Autodesk Inventor part; units mm, degrees
ref_plane "YZ Plane" through (0, 0, 0) normal (1, 0, 0) x (0, 1, 0)
ref_plane "XZ Plane" through (0, 0, 0) normal (0, 1, 0) x (-1, 0, 0)
ref_plane "XY Plane" through (0, 0, 0) normal (0, 0, 1) x (1, 0, 0)
sketch "Sketch1" plane through (0, 0, 0) normal (0, 1, 0) x (-1, 0, 0)
  line L0 (32.5791, 64.9096) -> (-50.4209, 64.9096)
  line L1 (-50.4209, 64.9096) -> (-50.4209, -78.0904)
  line L2 (-50.4209, -78.0904) -> (32.5791, -78.0904)
  line L3 (32.5791, -78.0904) -> (32.5791, 64.9096)
  line L4 (29.5791, 61.9096) -> (-47.4209, 61.9096)
  line L5 (-47.4209, 61.9096) -> (-47.4209, -75.0904)
  line L6 (-47.4209, -75.0904) -> (29.5791, -75.0904)
  line L7 (29.5791, -75.0904) -> (29.5791, 61.9096)
  line L8 (29.5791, -75.0904) -> (29.5791, -78.0904)
  line L9 (-47.4209, -70.2006) -> (-50.4209, -70.2006)
  line L10 (-47.4209, 33.4969) -> (-50.4209, 33.4969)
  line L11 (29.5791, 57.9608) -> (32.5791, 57.9608)
  line L12 (29.5791, -75.0904) -> (32.5791, -75.0904)
  point P0 (0, 0)
  dimension "d0" = 143
  dimension "d1" = 83
  dimension "d2" = 3
extrude "Floor" add sketch "Sketch1" along normal blind 3
extrude "Walls" add sketch "Sketch1" along normal blind 20 contours L3 L11 L7 L4 L5 L10 L1 L0 | L3 L12 L7 L11 | L10 L5 L9 L1 | L3 L2 L8 L12 | L9 L5 L6 L8 L2 L1
sketch "Sketch2" plane through (0, 0, 0) normal (0, 1, 0) x (-1, 0, 0)
  line L0 (-47.4209, 61.9096) -> (29.5791, 61.9096)
  line L1 (29.5791, -75.0904) -> (-47.4209, -75.0904)
  line L2 (29.5791, 61.9096) -> (29.5791, -75.0904)
  line L3 (-47.4209, -75.0904) -> (-47.4209, 61.9096)
  circle A0 centre (25.5791, 57.9096) radius 2.5
  circle A1 centre (-43.4209, 57.9096) radius 2.5
  circle A2 centre (-43.4209, -71.0904) radius 2.5
  circle A3 centre (-2.5209, -71.0904) radius 2.5
  line L4 (-47.4209, 61.9096) -> (-47.4209, -75.0904)
  line L5 (-47.4209, -68.5904) -> (-50.4209, -68.5904)
  line L6 (-50.4209, -68.5904) -> (-50.4209, 27.9367)
  line L7 (-50.4209, 64.9096) -> (-50.4209, -78.0904)
  line L8 (-47.4209, 27.9367) -> (-50.4209, 27.9367)
  line L9 (29.5791, -75.0904) -> (29.5791, 61.9096)
  line L10 (29.5791, 55.4096) -> (32.4454, 55.4096)
  line L11 (-47.4209, -75.0904) -> (29.5791, -75.0904)
  line L12 (29.5791, -75.0904) -> (29.5791, -78.0904)
  point P0 (0, 0)
  dimension "d30" = 4
  dimension "d31" = 4
  dimension "d32" = 4
  dimension "d33" = 4
  dimension "d34" = 4
  dimension "d35" = 4
  dimension "d36" = 4
  dimension "d37" = 32.1
extrude "mounts" add sketch "Sketch2" along normal blind 8 contours A0 | A1 | A2 | A3
hole "Hole1" at (43.4209, 0, -71.0904) at (43.4209, 0, 57.9096) at (2.5209, 0, -71.0904) at (-25.5791, 0, 57.9096) direction (0, 1, 0) diameter 3 depth 8
extrude "Extrusion5" cut sketch "Sketch1" along normal blind 20 contours L10 L5 L9 L1
extrude "Extrusion6" cut sketch "Sketch1" along normal blind 20 contours L3 L12 L7 L11 | L3 L2 L8 L12
extrude "Extrusion7" add sketch "Sketch1" along normal blind 8 contours L10 L5 L9 L1
extrude "Extrusion8" add sketch "Sketch1" along normal blind 8 contours L3 L12 L7 L11 | L3 L2 L8 L12
sketch "Sketch3" plane through (-32.5791, 0, 64.9096) normal (0, 0, 1) x (1, 0, 0)
  line L0 (0, 0) -> (0, 20) construction
  line L1 (0, 10) -> (97.9753, 10) construction
  line L2 (0, 20) -> (83, 20) construction
  line L3 (5.9967, 10) -> (23.1011, 10) construction
  line L4 (5.9967, 7.25) -> (23.1011, 7.25)
  line L5 (23.1011, 12.75) -> (5.9967, 12.75)
  arc A0 (5.9967, 12.75) -> (5.9967, 7.25) centre (5.9967, 10) ccw
  arc A1 (23.1011, 7.25) -> (23.1011, 12.75) centre (23.1011, 10) ccw
  line L6 (75.4862, 10) -> (58.3819, 10) construction
  line L7 (75.4862, 12.5) -> (58.3819, 12.5)
  line L8 (58.3819, 7.5) -> (75.4862, 7.5)
  arc A2 (75.4862, 7.5) -> (75.4862, 12.5) centre (75.4862, 10) ccw
  arc A3 (58.3819, 12.5) -> (58.3819, 7.5) centre (58.3819, 10) ccw
  line L9 (0, 0) -> (83, 0)
  point P0 (32.5791, 0)
  point P1 (14.5489, 10)
  point P2 (66.9341, 10)
  point P3 (40.0449, 10)
  dimension "d59" = 5.5
  dimension "d60" = 5
  dimension "d80" = 10
  dimension "d81" = 10
extrude "Extrusion9" add sketch "Sketch3" along normal blind 4.2
chamfer "Chamfer1" distance 1.25 angle 45 8 edges at (-6.7281, 10, 69.1096) (-18.0302, 12.75, 69.1096) (-29.3324, 10, 69.1096) (-18.0302, 7.25, 69.1096) (45.4071, 10, 69.1096) (34.3549, 12.5, 69.1096) (23.3027, 10, 69.1096) (34.3549, 7.5, 69.1096)
hole "Hole2" at (8.9209, 10, 64.9096) direction (0, 0, 1) diameter 4 depth 3
extrude "Extrusion10" add sketch "Sketch1" along normal blind 45 contours L3 L11 L7 L4 L5 L10 L1 L0
extrude "Extrusion11" add sketch "Sketch1" along normal blind 45 contours L9 L5 L6 L8 L2 L1
extrude "Extrusion12" add sketch "Sketch1" along normal blind 45 contours L3 L2 L8 L12
ref_plane "Work Plane1" through (47.4209, 45, -75.0904) normal (0, 1, 0) x (1, 0, 0)
sketch "Sketch4" plane through (0, 45, 0) normal (0, 1, 0) x (1, 0, 0)
  line L0 (47.4209, -61.9096) -> (47.4209, 75.0904)
  line L1 (47.4209, -61.9096) -> (38.4209, -61.9096)
  line L2 (38.4209, -61.9096) -> (38.4209, -52.9096)
  line L3 (38.4209, -52.9096) -> (47.4209, -52.9096)
  line L4 (47.4209, -52.9096) -> (47.4209, -61.9096)
  line L5 (47.4209, -61.9096) -> (-29.5791, -61.9096)
  line L6 (-29.5791, -61.9096) -> (-20.5791, -61.9096)
  line L7 (-20.5791, -61.9096) -> (-20.5791, -52.9096)
  line L8 (-20.5791, -52.9096) -> (-29.5791, -52.9096)
  line L9 (-29.5791, -52.9096) -> (-29.5791, -61.9096)
  line L10 (47.4209, 75.0904) -> (-29.5791, 75.0904)
  line L11 (47.4209, 75.0904) -> (38.4209, 75.0904)
  line L12 (38.4209, 75.0904) -> (38.4209, 66.0904)
  line L13 (38.4209, 66.0904) -> (47.4209, 66.0904)
  line L14 (47.4209, 66.0904) -> (47.4209, 75.0904)
  line L15 (-29.5791, 75.0904) -> (-20.5791, 75.0904)
  line L16 (-20.5791, 75.0904) -> (-20.5791, 66.0904)
  line L17 (-20.5791, 66.0904) -> (-29.5791, 66.0904)
  line L18 (-29.5791, 66.0904) -> (-29.5791, 75.0904)
  line L19 (-32.5791, 75.0904) -> (47.4209, 75.0904)
  point P0 (0, 0)
  dimension "d84" = 9
  dimension "d85" = 9
  dimension "d86" = 9
  dimension "d87" = 9
  dimension "d88" = 9
  dimension "d89" = 9
  dimension "d90" = 9
extrude "Extrusion13" add sketch "Sketch4" against normal blind 5 contours L5 L9 L8 L7
extrude "Extrusion14" add sketch "Sketch4" against normal blind 5 contours L1 L2 L3 L0 | L13 L12 L10 L0 | L16 L17 L18 L10
properties part number "rumba_frame_mount"
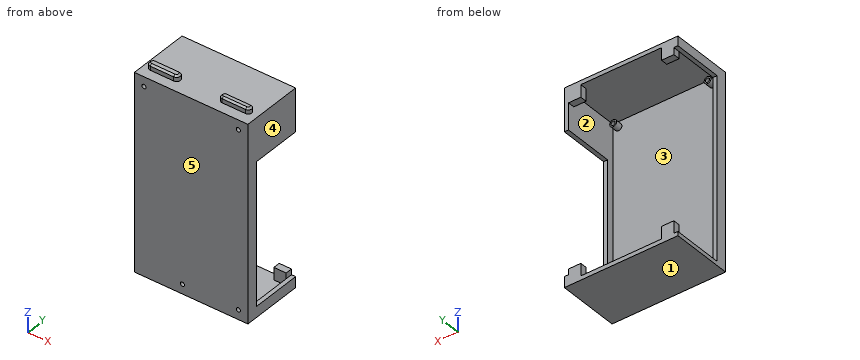
For this review, take the finished solid that the model builds, in its own axes (mm). Face numbers are marked on the shaded views. A direction names the side the tool comes from. Give positions to 0.01 mm unless a question says otherwise; leave off trailing zeros. Loops run counter-clockwise (first coordinate to the right, second up) from the corner with the lowest first, then second, coordinate; pieces in that order, holes last. Notation, with made-up numbers: M 43,-27 L 74,-27 A12 cw 74,-17 Z; hole C -7.5,57.5 d3. An arc over 180 degrees is marked long. Put each result on its own line as item: value. Start each with the question number.
(1) Add section D-D, the plane x = 35. Write out the cut boundary in (y, z).
(2) Add section C-C, the plane y = 5. Give the number of separate pieces and of enclosed holes in the cut face, then the cut area to 3 significant figures.
(3) Wall thickness on L1, parallel to X at y = 6.5, z = 6.5; L2, parallel to Z at x = 47.5, y = 17; L3, parallel to Z at x = -26.5, y = 8.5: over which ranges is each line inside the solid? List them lowest first.
(4) Add section A-A, the plane y = 23. Write out the cut boundary in (x, z).
(5) The part is to be moulded in two halves that separate along X. For the marked faces 3, 4 and 5, say which applies: +X half, -X half, draft (parallel to the pull), parting line (faces both ways), or undercut.
(6) For pin 1 (3 mm diameter, centred on x = 31, z = 66.5, fed in from +Y); pin 2 (2 mm diameter, centred on x = 21.5, y = 22.5, fed in from +Z); pin 3 (1.5 mm diameter, centred on x = -22, z = 66, fed in from +Y), all flat-tipped, find the tip position at first contact; note any pin that passes through.
(7) Machinability: for the marked faces 1 and 2, which of the approach directions +Z, -Z, +X, -X, +Y, -Y give a long, thin tool a straight path to every point of the face, cutting with its end or side? Answer none if there is none.
(8) Add section B-B, the plane z = -47.5. Write out the cut boundary in (x, y).
Result:
1. outline: M 0,-78.09 L 45,-78.09 L 45,-75.09 L 3,-75.09 L 3,61.91 L 45,61.91 L 45,64.91 L 12.5,64.91 L 12.5,67.86 L 11.25,69.11 L 8.75,69.11 L 7.5,67.86 L 7.5,64.91 L 0,64.91 Z
2. separate pieces: 5
2. enclosed holes: 5
2. area: 1,370 mm^2
3. L1: x = -32.58 to -29.58, 47.42 to 50.42
3. L2: z = -78.09 to -70.2, 33.5 to 64.91
3. L3: z = -78.09 to -75.09, 61.91 to 69.11
4. outline: M -32.58,-78.09 L 50.42,-78.09 L 50.42,-70.2 L 47.42,-70.2 L 47.42,-75.09 L -32.58,-75.09 Z; M -32.58,57.96 L -29.58,57.96 L -29.58,61.91 L 47.42,61.91 L 47.42,33.5 L 50.42,33.5 L 50.42,64.91 L -32.58,64.91 Z
5. face 3: undercut
5. face 4: +X half
5. face 5: draft
6. pin 1: stops at y = 12.5
6. pin 2: stops at z = 64.91
6. pin 3: stops at y = 12.75
7. face 1: -Z, +X, -X, +Y, -Y
7. face 2: none
8. outline: M -32.58,0 L 50.42,0 L 50.42,8 L 47.42,8 L 47.42,3 L -29.58,3 L -29.58,8 L -32.58,8 Z
